```python
from build123d import *
from build123d.topology import SkipClean

# Parameters (mm, degrees)
BASPROSKE_W         = 10
BASPROSKE_H         = 10.625
TOOTHCUT_DEPTH      = 19.049411348
TEETHCUTS_COUNT     = 15
TEETHCUTS_ANGLE     = 336
BORSKE_R            = 1.5
BORE_DEPTH          = 50.0000508
BOSS_EXTRUDE1_START = 10
SKETCH1_R           = 7.8115
SKETCH1_R_2         = 1.5
BOSS_EXTRUDE1_DEPTH = 10
BOSS_EXTRUDE2_DEPTH = 20


with BuildPart() as part:
    # BasProSke → Base-Revolve (revolve)
    with BuildSketch(Plane(origin=(0, 0, 0), x_dir=(1, 0, 0), z_dir=(0, 1, 0)), mode=Mode.PRIVATE) as base_revolve_sk:
        with Locations((5, 5.3125)):
            Rectangle(BASPROSKE_W, BASPROSKE_H)
    revolve(base_revolve_sk.sketch.rotate(Axis((-10, 0, 0), (1, 0, 0)), 180), axis=Axis((-10, 0, 0), (1, 0, 0)))

    # TooCutSke → ToothCut (cut, through all)
    with BuildSketch(Plane(origin=(0, 0, 0), x_dir=(0, 0, -1), z_dir=(1, 0, 0))):
        with BuildLine():
            ThreePointArc((0.660831632, 7.78349753), (0, 7.8115), (-0.660831632, 7.78349753))
            ThreePointArc((-0.660831632, 7.78349753), (-1.031814994, 9.260718016), (-1.959681305, 10.46855622))
            ThreePointArc((-1.959681305, 10.46855622), (0, 10.6504), (1.959681305, 10.46855622))
            ThreePointArc((1.959681305, 10.46855622), (1.031814994, 9.260718016), (0.660831632, 7.78349753))
        make_face()
    toothcut = extrude(amount=TOOTHCUT_DEPTH, mode=Mode.SUBTRACT)

    # TeethCuts: ToothCut ×15 about axis
    teethcuts_axis = Axis((-10, 0, 0), (1, 0, 0))
    for i in range(1, TEETHCUTS_COUNT):
        add(toothcut.rotate(teethcuts_axis, i * TEETHCUTS_ANGLE / (TEETHCUTS_COUNT - 1)), mode=Mode.SUBTRACT)

    # BorSke → Bore (cut, symmetric)
    with BuildSketch(Plane(origin=(0, 0, 0), x_dir=(0, 0, -1), z_dir=(1, 0, 0))):
        with Locations(Location((0, 0, 0), (0, 0, 180))):
            Circle(BORSKE_R)
    extrude(amount=BORE_DEPTH, both=True, mode=Mode.SUBTRACT)

    # Sketch1 → Boss-Extrude1 (add)
    with SkipClean():  # the faces are left unmerged after this step: merging them gives an invalid solid
        with BuildSketch(Plane.ZY.offset(BOSS_EXTRUDE1_START)):
            Circle(SKETCH1_R)
            Circle(SKETCH1_R_2, mode=Mode.SUBTRACT)
        extrude(amount=-BOSS_EXTRUDE1_DEPTH)

    # Sketch2 → Boss-Extrude2 (add)
    with SkipClean():  # the faces are left unmerged after this step: merging them gives an invalid solid
        with BuildSketch(Plane(origin=(10, 0, 0), x_dir=(0, 0, -1), z_dir=(1, 0, 0))):
            with BuildLine():
                ThreePointArc((0.739577582, 1.305), (0, 1.5), (-0.739577582, 1.305))
                Line((-0.739577582, 1.305), (0.739577582, 1.305))
            make_face()
        extrude(amount=-BOSS_EXTRUDE2_DEPTH)


solid = part.part
```
Work out the finished part from the listing and answer in its coordinate system (mm). A direction names the side the tool comes from. Round coordinates to 2 decimals unless told otherwise and drop trailing zeros. Loops run counter-clockwise (first coordinate to the right, second up) from the corner with the lowest first, then second, coordinate; pieces in that order, holes last. Notation, with made-up numbers: (-30, -25.5) -> (23, -25.5) arc R20 cw to (23, -9.5) -> close; hole circle Ø5 at (63, 3.5). An arc over 180 degrees is marked (long way). Write each question's results on one line, items separated by ' | '. Start each with the question number.
1. Given pin 1 Ø10 at (x, y) = (-6, -3.5) entering from -Z; pin 2 Ø1.3 at (y, z) = (3.5, -8.5) entering from -X; pin 3 Ø5 at (x, z) = (1, -4.5) entering from +Y, each flat-ended and moving along its own axis, determine where each tip first touches the part or whether it passes through.
2. A tool of negligible diameter and unlimited length cuts with its end or side. For faces 1 (the face through (4.93, 6.968, 6.194)), 2 (the face through (4.93, -9.236, 0.925)), 3 (the face through (4.9, -8.8, 2.9)), 4 (the face through (0, -8, -4)), from which of +Z, -Z, +X, -X, +Y, -Y can it reach the whole face along a straight path? Write none if from no direction.
3. Section C-C (z = 3.25) is taken. Determine the outline of the cut face in (x, y).
4. Section B-B (x = -7.25) is taken. Determine the outline of the cut face in (y, z) (1 decimal).
5. Section A-A (y = -1) is taken. Determine the outline of the cut face in (x, z).
6. For a pull along Y with two mould halves and no side action, classify faces 5 (the face through (4.93, -5.53, -7.51)), 6 (the face through (0, 9, 2)), 7 (the face through (4.93, -6.87, -6.25)) as +Y half, -Y half, draft (parallel to the pull), parting line (faces both ways), or undercut.
7. Find the intervals of material crossed by probe 1 along Z at (x, y) = (-1.5, 0); probe 2 along X at (y, z) = (-8.25, 4); probe 3 along Z at (x, y) = (5.25, 0.75), in increasing order. Write a range as from..to.
8. Section D-D (y = 6) is taken. Determine the outline of the cut face in (x, z), plus the area to 3 significant figures.
Evaluation:
1) pin 1: stops at z = -7.81 | pin 2: stops at x = 0 | pin 3: stops at y = 10.44
2) face 1: +Z, +X, -X | face 2: +X, -X | face 3: +X, -X, -Y | face 4: -Z, -X, -Y
3) outline: (-10, -7.1) -> (0, -7.1) -> (0, -9.2) -> (10, -9.2) -> (10, 7.1) -> (-10, 7.1) -> close
4) outline: circle Ø15.6 at (0, 0); hole (1.3, -0.7) -> (1.3, 0.7) arc R1.5 ccw (long way) to start
5) outline: (-10, -7.75) -> (10, -7.75) -> (10, -1.12) -> (-10, -1.12) -> close; (-10, 1.12) -> (10, 1.12) -> (10, 7.75) -> (-10, 7.75) -> close
6) face 5: undercut | face 6: draft | face 7: -Y half
7) probe 1: z = -7.81..-1.5, 1.5..7.81 | probe 2: x = 0..10 | probe 3: z = -10.5..-1.3, 1.3..10.5
8) outline: (-10, -5) -> (0, -5) -> (0, -5.62) -> (10, -5.62) -> (10, 5.62) -> (0, 5.62) -> (0, 5) -> (-10, 5) -> close | area: 212 mm2
